```python
from build123d import *

# Parameters (mm, degrees)
BOSS_EXTRUDE2_DEPTH = 3.175
BOSS_EXTRUDE3_DEPTH = 3.175
SKETCH11_W          = 113.03
SKETCH11_H          = 79.94142
BOSS_EXTRUDE8_DEPTH = 3.175
SKETCH12_W          = 70.49262
SKETCH12_H          = 3.175
BOSS_EXTRUDE9_DEPTH = 3.175
SKETCH15_R          = 2.25
CUT_EXTRUDE1_DEPTH  = 371.49176257
SKETCH16_R          = 2.250000072
SKETCH16_R_2        = 2.25
CUT_EXTRUDE2_DEPTH  = 371.49176257
SKETCH17_R          = 5
CUT_EXTRUDE3_DEPTH  = 371.49176257


with BuildPart() as part:
    # Sketch1 → Boss-Extrude2 (new body)
    with BuildSketch(Plane.XY):
        Polygon((129.013076168, 254.245404572), (-18.685383832, 254.245404572), (-18.685383832, 157.666984572), (92.088461168, 157.666984572), (92.088461168, 154.491984572), (-18.685383832, 154.491984572), (-18.685383832, 57.913564572), (92.088461168, 57.913564572), (92.088461168, 54.738564572), (-18.685383832, 54.738564572), (-18.685383832, -41.839855428), (92.088461168, -41.839855428), (92.088461168, -45.014855428), (-18.685383832, -45.014855428), (-18.685383832, -141.593275428), (92.088461168, -141.593275428), (92.088461168, -144.768275428), (-18.685383832, -144.768275428), (-18.685383832, -241.346695428), (129.013076168, -241.346695428), align=None)
    extrude(amount=BOSS_EXTRUDE2_DEPTH)

    # Sketch4 → Boss-Extrude3 (add, through all)
    with BuildSketch(Plane.XY.offset(3.175)):
        Polygon((129.013076168, 254.245404572), (129.013076168, -241.346695428), (153.407236168, -241.346695428), (153.407236168, -227.262720585), (153.407236168, 240.16142973), (153.407236168, 254.245404572), align=None)
    extrude(amount=-BOSS_EXTRUDE3_DEPTH)

    # Sketch11 → Boss-Extrude8 (add, through all)
    with BuildSketch(Plane.XY.offset(3.175)):
        with Locations((209.922236168, 94.709274572)):
            Rectangle(SKETCH11_W, SKETCH11_H)
    extrude(amount=-BOSS_EXTRUDE8_DEPTH)

    # Sketch12 → Boss-Extrude9 (add, through all)
    with BuildSketch(Plane(origin=(0, 0, 0), x_dir=(-1, 0, 0), z_dir=(0, 0, -1))):
        with Locations((-16.560926168, 255.832904572)):
            Rectangle(SKETCH12_W, SKETCH12_H)
        with Locations((-16.560926168, -242.934195428)):
            Rectangle(SKETCH12_W, SKETCH12_H)
    extrude(amount=-BOSS_EXTRUDE9_DEPTH)

    # Sketch15 → Cut-Extrude1 (cut, through all)
    with BuildSketch(Plane.XY.offset(3.175)):
        with Locations((143.247236168, 231.313297791)):
            Circle(SKETCH15_R)
        with Locations((143.247236168, 164.651984572)):
            Circle(SKETCH15_R)
        with Locations((255.799716168, 113.343984572)):
            Circle(SKETCH15_R)
        with Locations((255.799716168, 74.495671354)):
            Circle(SKETCH15_R)
        with Locations((143.247236168, 29.338564572)):
            Circle(SKETCH15_R)
        with Locations((143.247236168, -32.334232694)):
            Circle(SKETCH15_R)
        with Locations((143.247236168, -94.538012037)):
            Circle(SKETCH15_R)
        with Locations((143.247236168, -156.74179138)):
            Circle(SKETCH15_R)
        with Locations((143.247236168, -218.414588646)):
            Circle(SKETCH15_R)
    extrude(amount=-CUT_EXTRUDE1_DEPTH, mode=Mode.SUBTRACT)

    # Sketch16 → Cut-Extrude2 (cut, through all)
    with BuildSketch(Plane.XY.offset(3.175)):
        with Locations((138.792076168, 121.451235566)):
            Circle(SKETCH16_R)
        with Locations((138.792076168, 82.140925566)):
            Circle(SKETCH16_R_2)
    extrude(amount=-CUT_EXTRUDE2_DEPTH, mode=Mode.SUBTRACT)

    # Sketch17 → Cut-Extrude3 (cut, through all)
    with BuildSketch(Plane.XY.offset(3.175)):
        with Locations((79.191467271, 4.016944877)):
            Circle(SKETCH17_R)
        with Locations((66.491467271, 4.016944877)):
            Circle(SKETCH17_R)
        with Locations((53.791467271, 4.016944877)):
            Circle(SKETCH17_R)
        with Locations((41.091467271, 4.016944877)):
            Circle(SKETCH17_R)
        with Locations((66.491467271, -7.413055123)):
            Circle(SKETCH17_R)
        with Locations((53.791467271, -7.413055123)):
            Circle(SKETCH17_R)
        with Locations((41.091467271, -7.413055123)):
            Circle(SKETCH17_R)
        with Locations((79.191467271, -7.413055123)):
            Circle(SKETCH17_R)
        with Locations(Location((41.091467271, -35.281788831, 0), (0, 0, 180))):
            Circle(SKETCH17_R)
        with Locations(Location((41.091467271, -23.851788831, 0), (0, 0, 180))):
            Circle(SKETCH17_R)
        with Locations(Location((53.791467271, -35.281788831, 0), (0, 0, 180))):
            Circle(SKETCH17_R)
        with Locations(Location((53.791467271, -23.851788831, 0), (0, 0, 180))):
            Circle(SKETCH17_R)
        with Locations(Location((66.491467271, -35.281788831, 0), (0, 0, 180))):
            Circle(SKETCH17_R)
        with Locations(Location((66.491467271, -23.851788831, 0), (0, 0, 180))):
            Circle(SKETCH17_R)
        with Locations(Location((79.191467271, -23.851788831, 0), (0, 0, 180))):
            Circle(SKETCH17_R)
        with Locations(Location((79.191467271, -35.281788831, 0), (0, 0, 180))):
            Circle(SKETCH17_R)
        with Locations((79.191467271, -195.489895123)):
            Circle(SKETCH17_R)
        with Locations((66.491467271, -195.489895123)):
            Circle(SKETCH17_R)
        with Locations((53.791467271, -195.489895123)):
            Circle(SKETCH17_R)
        with Locations((41.091467271, -195.489895123)):
            Circle(SKETCH17_R)
        with Locations((66.491467271, -206.919895123)):
            Circle(SKETCH17_R)
        with Locations((53.791467271, -206.919895123)):
            Circle(SKETCH17_R)
        with Locations((41.091467271, -206.919895123)):
            Circle(SKETCH17_R)
        with Locations((79.191467271, -206.919895123)):
            Circle(SKETCH17_R)
        with Locations(Location((41.091467271, -234.788628831, 0), (0, 0, 180))):
            Circle(SKETCH17_R)
        with Locations(Location((41.091467271, -223.358628831, 0), (0, 0, 180))):
            Circle(SKETCH17_R)
        with Locations(Location((53.791467271, -234.788628831, 0), (0, 0, 180))):
            Circle(SKETCH17_R)
        with Locations(Location((53.791467271, -223.358628831, 0), (0, 0, 180))):
            Circle(SKETCH17_R)
        with Locations(Location((66.491467271, -234.788628831, 0), (0, 0, 180))):
            Circle(SKETCH17_R)
        with Locations(Location((66.491467271, -223.358628831, 0), (0, 0, 180))):
            Circle(SKETCH17_R)
        with Locations(Location((79.191467271, -223.358628831, 0), (0, 0, 180))):
            Circle(SKETCH17_R)
        with Locations(Location((79.191467271, -234.788628831, 0), (0, 0, 180))):
            Circle(SKETCH17_R)
        with Locations((79.191467271, 175.728851427)):
            Circle(SKETCH17_R)
        with Locations((66.491467271, 175.728851427)):
            Circle(SKETCH17_R)
        with Locations((53.791467271, 175.728851427)):
            Circle(SKETCH17_R)
        with Locations((41.091467271, 175.728851427)):
            Circle(SKETCH17_R)
        with Locations((66.491467271, 164.298851427)):
            Circle(SKETCH17_R)
        with Locations((53.791467271, 164.298851427)):
            Circle(SKETCH17_R)
        with Locations((41.091467271, 164.298851427)):
            Circle(SKETCH17_R)
        with Locations((79.191467271, 164.298851427)):
            Circle(SKETCH17_R)
        with Locations(Location((41.091467271, 136.430117718, 0), (0, 0, 180))):
            Circle(SKETCH17_R)
        with Locations(Location((41.091467271, 147.860117718, 0), (0, 0, 180))):
            Circle(SKETCH17_R)
        with Locations(Location((53.791467271, 136.430117718, 0), (0, 0, 180))):
            Circle(SKETCH17_R)
        with Locations(Location((53.791467271, 147.860117718, 0), (0, 0, 180))):
            Circle(SKETCH17_R)
        with Locations(Location((66.491467271, 136.430117718, 0), (0, 0, 180))):
            Circle(SKETCH17_R)
        with Locations(Location((66.491467271, 147.860117718, 0), (0, 0, 180))):
            Circle(SKETCH17_R)
        with Locations(Location((79.191467271, 147.860117718, 0), (0, 0, 180))):
            Circle(SKETCH17_R)
        with Locations(Location((79.191467271, 136.430117718, 0), (0, 0, 180))):
            Circle(SKETCH17_R)
    extrude(amount=-CUT_EXTRUDE3_DEPTH, mode=Mode.SUBTRACT)


solid = part.part
```
Build history of the part. All positions in model axes, mm. Round coordinates to 2 decimals unless told otherwise and drop trailing zeros. Loops run counter-clockwise (first coordinate to the right, second up) from the corner with the lowest first, then second, coordinate; pieces in that order, holes last. Notation, with made-up numbers: M -38,-13 L -2,-13 A16 ccw -2,-7 Z; hole C -4.75,4 d9. An arc over 180 degrees is marked long. Answer as CSV lines item,"result".
1. Two-plate mould, pull along X, no slides. Class faces 1 (the flat face through (94, 10, 3.175)), 2 (the cylindrical face through (52.708, 159.418, 1.61)): released by +X, released by -X, zero draft, split by the parting line, or undercut.
Resolved:
face 1,"zero draft"
face 2,"undercut"
2. Flat gauge pins, fed straight in: P1, Ø9, axis at x = 53.79, y = 164.3, coming from the -Z side; P2, Ø1, axis at y = 56.5, z = 1, coming from the -X side. Where does each tip first touch, or does it go through?
Resolved:
P1,"passes through"
P2,"stops at x = 92.09"
3. Cut at B-B on z = 0.6. Count the separate pieces of the cut face and the enclosed holes in it, then the cut area to 3 significant figures.
Resolved:
separate pieces,"1"
enclosed holes,"59"
area,"89,400 mm²"
4. Wall check: probe 1 along Y at (x, z) = (1.5, 3); probe 2 along X at (y, z) = (176.5, 2.45); probe 3 along X at (y, z) = (-84.5, 0.35). Give the ranges that are in metal, low to high. Write a range as [from, to].
Resolved:
probe 1,"y = [-244.52, -144.77], [-141.59, -45.01], [-41.84, 54.74], [57.91, 154.49], [157.67, 257.42]"
probe 2,"x = [-18.69, 36.15], [46.03, 48.85], [58.73, 61.55], [71.43, 74.25], [84.13, 153.41]"
probe 3,"x = [-18.69, 153.41]"
5. Cut at A-A on x = 209. Write the cut outline in (y, z) (3 decimals).
Resolved:
outline,"M 54.739,0 L 134.68,0 L 134.68,3.175 L 54.739,3.175 Z"
